Input: part model. Units: mm. Frame: model coordinates. A direction names the side the tool comes from. Give positions to 0.01 mm unless a question says otherwise; leave off trailing zeros. Loops run counter-clockwise (first coordinate to the right, second up) from the corner with the lowest first, then second, coordinate; pieces in that order, holes last. Notation, with made-up numbers: (33, 79.5) -> (75, 79.5) arc R14 ccw to (75, 96.5) -> close; hole circle Ø6 at (27, 74.5). An arc over 180 degrees is marked (long way). Answer as a JSON object with one key per item and string values. Group by question number.
```python
from build123d import *

# Parameters (mm, degrees)
BOSS_EXTRUDE1_DEPTH = 35
SKETCH5_R           = 1.905
CUT_EXTRUDE1_DEPTH  = 35
SKETCH2_R           = 1.905
CUT_EXTRUDE2_DEPTH  = 49.85
SKETCH7_W           = 11
SKETCH7_H           = 1.5
BOSS_EXTRUDE3_DEPTH = 1.5
SKETCH8_R           = 1.905
CUT_EXTRUDE3_DEPTH  = 49.85
SKETCH11_R          = 3.25
SKETCH11_R_2        = 1.905
BOSS_EXTRUDE4_DEPTH = 13.3


with BuildPart() as part:
    # Sketch1 → Boss-Extrude1 (new body)
    with BuildSketch(Plane.XY):
        Polygon((0, 0), (13, 0), (13, 34), (13, 49), (0, 49), (0, 34), (-35.85, 34), (-35.85, 30), (0, 30), align=None)
    extrude(amount=-BOSS_EXTRUDE1_DEPTH)

    # Sketch5 → Cut-Extrude1 (cut, through all)
    with BuildSketch(Plane(origin=(0, 34, 0), x_dir=(1, 0, 0), z_dir=(0, 1, 0))):
        with Locations((-31.25, 4.8)):
            Circle(SKETCH5_R)
        with Locations((-31.25, 30.2)):
            Circle(SKETCH5_R)
    extrude(amount=-CUT_EXTRUDE1_DEPTH, mode=Mode.SUBTRACT)

    # Sketch2 → Cut-Extrude2 (cut, through all)
    with BuildSketch(Plane(origin=(13, 0, 0), x_dir=(0, 0, -1), z_dir=(1, 0, 0))):
        with Locations((4.8, 4.1)):
            Circle(SKETCH2_R)
        with Locations((30.2, 4.1)):
            Circle(SKETCH2_R)
    extrude(amount=-CUT_EXTRUDE2_DEPTH, mode=Mode.SUBTRACT)

    # Sketch7 → Boss-Extrude3 (add)
    with BuildSketch(Plane(origin=(13, 0, 0), x_dir=(0, 0, -1), z_dir=(1, 0, 0))):
        with Locations((17.5, 8.75)):
            Rectangle(SKETCH7_W, SKETCH7_H)
    extrude(amount=BOSS_EXTRUDE3_DEPTH)

    # Sketch8 → Cut-Extrude3 (cut, through all)
    with BuildSketch(Plane(origin=(13, 0, 0), x_dir=(0, 0, -1), z_dir=(1, 0, 0))):
        with Locations((4.8, 44.1)):
            Circle(SKETCH8_R)
        with Locations((30.2, 44.1)):
            Circle(SKETCH8_R)
    extrude(amount=-CUT_EXTRUDE3_DEPTH, mode=Mode.SUBTRACT)

    # Sketch11 → Boss-Extrude4 (add)
    with BuildSketch(Plane(origin=(13, 0, 0), x_dir=(0, 0, -1), z_dir=(1, 0, 0))):
        with Locations((4.8, 44.1)):
            Circle(SKETCH11_R)
        with Locations((4.8, 44.1)):
            Circle(SKETCH11_R_2, mode=Mode.SUBTRACT)
        with Locations((30.2, 44.1)):
            Circle(SKETCH11_R)
        with Locations((30.2, 44.1)):
            Circle(SKETCH11_R_2, mode=Mode.SUBTRACT)
        with Locations((30.2, 4.1)):
            Circle(SKETCH11_R)
        with Locations((30.2, 4.1)):
            Circle(SKETCH11_R_2, mode=Mode.SUBTRACT)
        with Locations((4.8, 4.1)):
            Circle(SKETCH11_R)
        with Locations((4.8, 4.1)):
            Circle(SKETCH11_R_2, mode=Mode.SUBTRACT)
    extrude(amount=BOSS_EXTRUDE4_DEPTH)


solid = part.part
```
Q1. Pin query (flat end, axial travel): pin 1 Ø1 at (x, z) = (-11, -8.5) entering from -Y; pin 2 Ø4.5 at (y, z) = (44.1, -30.2) entering from +X; pin 3 Ø1.2 at (x, z) = (14, -19) entering from -Y; pin 4 Ø1.2 at (y, z) = (8.5, -18.5) entering from +X. Return the tip coordinate at first contact, or that it passes through.
Q2. Set-up query: faces 1 (the face through (14, 8, -17)), 2 (the face through (19.56, 45.08, -7.9)), 3 (the face through (14, 9, -23)), 4 (the face through (14, 9, -12)), 5 (the face through (0, 15, -17)). Return all of +Z, -Z, +X, -X, +Y, -Y with unobstructed straight access to the full face (end or side cutting, diameter ignored); none if empty.
Q3. Section A-A on y = 44.1. Return the cut outline in (x, z) (3 decimals).
Q4. Section D-D on y = 26. Return the cut outline in (x, z).
Q5. Section B-B on z = -30.2. Return the cut outline in (x, y) (3 decimals), then the cut area to 3 significant figures.
Q6. Section C-C on z = -24.5. Return the cut outline in (x, y).
Q7. Pull-direction query (Y, two-part tool) for faces 6 (the face through (-18, 30, -17)), 7 (the face through (14, 9.5, -17)), 8 (the face through (19.557, 4.243, -26.953)); classes: +Y half, -Y half, draft (parallel to the pull), parting line (faces both ways), or undercut.
Q8. Ray query, probe 1 along Z at (x, y) = (17, 44); probe 2 along Z at (x, y) = (-31.25, 32.65) (3 decimals); probe 3 along Y at (x, z) = (7, -4.8) (3 decimals). Return the intervals inside material, ascending.
Numbers:
{
 "1": {"pin 1": "stops at y = 30", "pin 2": "stops at x = 26.3", "pin 3": "stops at y = 8", "pin 4": "stops at x = 14.5"},
 "2": {"face 1": "+Z, -Z, +X, -Y", "face 2": "+X", "face 3": "-Z, +X, +Y, -Y", "face 4": "+Z, +X, +Y, -Y", "face 5": "+Z, -Z, -X, -Y"},
 "3": {"outline": "(0, -35) -> (13, -35) -> (13, -33.45) -> (26.3, -33.45) -> (26.3, -32.105) -> (0, -32.105) -> close; (0, -28.295) -> (26.3, -28.295) -> (26.3, -26.95) -> (13, -26.95) -> (13, -8.05) -> (26.3, -8.05) -> (26.3, -6.705) -> (0, -6.705) -> close; (0, -2.895) -> (26.3, -2.895) -> (26.3, -1.55) -> (13, -1.55) -> (13, 0) -> (0, 0) -> close"},
 "4": {"outline": "(0, -35) -> (13, -35) -> (13, 0) -> (0, 0) -> close"},
 "5": {"outline": "(-35.85, 30) -> (-33.155, 30) -> (-33.155, 34) -> (-35.85, 34) -> close; (-29.345, 30) -> (0, 30) -> (0, 6.005) -> (26.3, 6.005) -> (26.3, 7.35) -> (13, 7.35) -> (13, 40.85) -> (26.3, 40.85) -> (26.3, 42.195) -> (0, 42.195) -> (0, 34) -> (-29.345, 34) -> close; (0, 0) -> (13, 0) -> (13, 0.85) -> (26.3, 0.85) -> (26.3, 2.195) -> (0, 2.195) -> close; (0, 46.005) -> (26.3, 46.005) -> (26.3, 47.35) -> (13, 47.35) -> (13, 49) -> (0, 49) -> close", "area": "738 mm²"},
 "6": {"outline": "(-35.85, 30) -> (0, 30) -> (0, 0) -> (13, 0) -> (13, 49) -> (0, 49) -> (0, 34) -> (-35.85, 34) -> close"},
 "7": {"face 6": "-Y half", "face 7": "+Y half", "face 8": "undercut"},
 "8": {"probe 1": "z = -33.45 to -32.1, -28.3 to -26.95, -8.05 to -6.7, -2.9 to -1.55", "probe 2": "z = -35 to -32.105, -28.295 to -6.705, -2.895 to 0", "probe 3": "y = 0 to 2.195, 6.005 to 42.195, 46.005 to 49"}
}
